Source: CAD feature listing. Evaluate the final solid. Frame: model axes, mm. A direction names the side the tool comes from. Give positions to 0.01 mm unless a question says otherwise; leave off trailing zeros. Order: outer loops, then holes, each group sorted by start corner. A loop starts at its lowest first (then second) coordinate and runs counter-clockwise, first axis right, second up.
from build123d import *

# Parameters (mm, degrees)
BOSS_EXTRU_1_DEPTH      = 404
ENL_V_MAT_EXTRU_1_DEPTH = 590
ENL_V_MAT_EXTRU_2_DEPTH = 590
ENL_V_MAT_EXTRU_3_DEPTH = 41
ENL_V_MAT_EXTRU_4_DEPTH = 41


with BuildPart() as part:
    # Esquisse1 → Boss.-Extru.1 (new body)
    with BuildSketch(Plane(origin=(0, 0, 0), x_dir=(1, 0, 0), z_dir=(0, 1, 0))):
        Polygon((-20, 20.113636364), (20, 20.113636364), (20, 18.113636364), (-18, 18.113636364), (-18, -19.886363636), (-20, -19.886363636), align=None)
    extrude(amount=BOSS_EXTRU_1_DEPTH)

    # Esquisse2 → Enlèv. mat.-Extru.1 (cut)
    with BuildSketch(Plane(origin=(0, 0, -20.113636364), x_dir=(-1, 0, 0), z_dir=(0, 0, -1))):
        Polygon((20, 0), (-20, 40), (-20, 0), align=None)
    extrude(amount=-ENL_V_MAT_EXTRU_1_DEPTH, mode=Mode.SUBTRACT)

    # Esquisse3 → Enlèv. mat.-Extru.2 (cut)
    with BuildSketch(Plane.ZY.offset(20)):
        Polygon((-20.113636364, 0), (19.886363636, 40), (19.886363636, 0), align=None)
    extrude(amount=-ENL_V_MAT_EXTRU_2_DEPTH, mode=Mode.SUBTRACT)

    # Esquisse4 → Enlèv. mat.-Extru.3 (cut, through all)
    with BuildSketch(Plane.ZY.offset(20)):
        Polygon((-20.113636364, 404), (19.886363636, 364), (19.886363636, 404), align=None)
    extrude(amount=-ENL_V_MAT_EXTRU_3_DEPTH, mode=Mode.SUBTRACT)

    # Esquisse5 → Enlèv. mat.-Extru.4 (cut, through all)
    with BuildSketch(Plane(origin=(0, 0, -20.113636364), x_dir=(-1, 0, 0), z_dir=(0, 0, -1))):
        Polygon((20, 404), (-20, 364), (-20, 404), align=None)
    extrude(amount=-ENL_V_MAT_EXTRU_4_DEPTH, mode=Mode.SUBTRACT)


solid = part.part
1) Reachability of faces 1 (the face through (-20, 199, 0)), 2 (the face through (-18, 199, 1)) from +Z, -Z, +X, -X, +Y, -Y: full face, straight path, thin tool, end or side. Return the list, or none.
Checks:
face 1: +Z, -Z, -X, +Y, -Y
face 2: +Z, +X, +Y, -Y
2) Section query D-D on y = 30. Output: boundary loops of the cut face in (x, z), and give its area (3 significant figures).
Checks:
outline: (-20, -20.11) - (10, -20.11) - (10, -18.11) - (-18, -18.11) - (-18, 9.89) - (-20, 9.89) - close
area: 116 mm2
3) Section query C-C on z = -5. Output: boundary loops of the cut face in (x, y), and give its area (3 significant figures).
Checks:
outline: (-20, 15.11) - (-18, 15.11) - (-18, 388.89) - (-20, 388.89) - close
area: 748 mm2
4) Ray query, L1, parallel to Z at x = -14, y = 28; L2, parallel to X at y = 297.5, z = -14. Return the intervals inside material, ascending.
Checks:
L1: z = -20.11 to -18.11
L2: x = -20 to -18
5) Section query B-B on x = 8.5. Output: boundary loops of the cut face in (y, z), and give its area (3 significant figures).
Checks:
outline: (28.5, -20.11) - (375.5, -20.11) - (375.5, -18.11) - (28.5, -18.11) - close
area: 694 mm2
6) Section query A-A on y = 83. Output: boundary loops of the cut face in (x, z).
Checks:
outline: (-20, -20.11) - (20, -20.11) - (20, -18.11) - (-18, -18.11) - (-18, 19.89) - (-20, 19.89) - close
7) First-contact query: pin 1 Ø3 at (x, y) = (-14.5, 113) entering from +Z; pin 2 Ø10 at (y, z) = (68.5, 12) entering from +X; pin 3 Ø12 at (x, z) = (6, -14.5) entering from -Y; pin 4 Ø8 at (y, z) = (316, -15.5) entering from +X. Flat tips, straight axial feed; report the tip coordinate or a pass-through.
Checks:
pin 1: stops at z = -18.11
pin 2: stops at x = -18
pin 3: stops at y = 21.21
pin 4: stops at x = 20
